Verification items for this drawing (mm, ordinates from the low corner). A direction names the side the tool comes from. Coordinates: 2 decimals unless noted, no trailing zeros. Order: outer loops, then holes, each group sorted by start corner. A loop starts at its lowest first (then second) coordinate and runs counter-clockwise, first axis right, second up. Notation, with made-up numbers: M -37,-32 L -19,-32 A20 ccw -19,-20 Z; hole C 10.5,67.25 d2. An arc over 180 degrees is marked long. Return JSON: item names as keys, results as strings. Group by question number.
1. Gauge pin test, flat ends, axial feed: pin 1 (1.8 mm diameter, centred on x = 7.5, y = 6.5, fed in from -Z); pin 2 (7 mm diameter, centred on y = 5.5, z = 6.5, fed in from +X); pin 3 (1 mm diameter, centred on x = 7.5, y = 2, fed in from -Z); pin 4 (1 mm diameter, centred on x = 9.5, y = 9, fed in from +Z) (1 decimal). Record the tip position at first contact, or that the pin passes through.
2. Section check A-A, the plane x = 7. Record the cut outline in (y, z) (1 decimal).
3. Section check B-B, the plane x = 9.5. Record the cut outline in (y, z) (1 decimal), plus the area to 3 significant figures.
4. Section check C-C, the plane x = 2.5. Record the cut outline in (y, z).
5. Material ranges on line 1 along Z through (x, y) = (10.25, 7.75) (1 decimal); line 2 along Z through (x, y) = (5.75, 6) (1 decimal); line 3 along X through (y, z) = (9, 5.5), recorded low to high.
6. Set-up check for the marked faces 1, 2 and 3: record each of +Z, -Z, +X, -X, +Y, -Y from which the full face is reachable in a straight line by a thin tool's end or side.
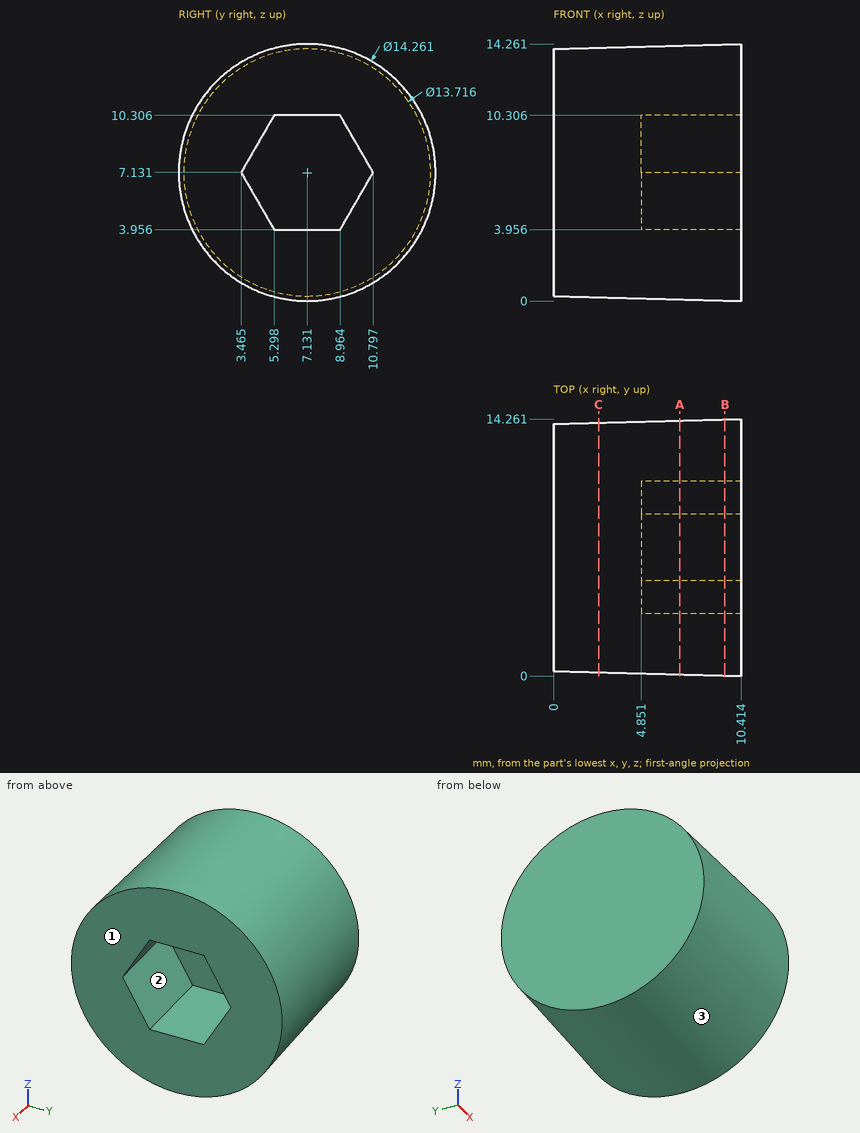
Answers follow:
{
 "1": {"pin 1": "z = 0.06", "pin 2": "x = 10.41", "pin 3": "z = 1.81", "pin 4": "z = 14.1"},
 "2": {"outline": "C 7.1,7.1 d14.1; hole M 3.5,7.1 L 5.3,4 L 9,4 L 10.8,7.1 L 9,10.3 L 5.3,10.3 Z"},
 "3": {"outline": "C 7.1,7.1 d14.2; hole M 3.5,7.1 L 5.3,4 L 9,4 L 10.8,7.1 L 9,10.3 L 5.3,10.3 Z", "area": "124 mm^2"},
 "4": {"outline": "C 7.13,7.13 d13.85"},
 "5": {"line 1": "0 to 4, 10.3 to 14.2", "line 2": "0.2 to 4, 10.3 to 14", "line 3": "0 to 4.85"},
 "6": {"face 1": "+Z, -Z, +X, +Y, -Y", "face 2": "+X", "face 3": "-X"}
}
